Answer from the drawing. Dimensions are ordinates in mm from the lowest x, y and z of the part. A direction names the side the tool comes from. Coordinates: 2 decimals unless noted, no trailing zeros. Loops run counter-clockwise (first coordinate to the right, second up) from the corner with the lowest first, then second, coordinate; pieces in that order, holes last. Notation, with made-up numbers: M 18,-3 L 70,-3 A25 cw 70,19 Z; hole C 63,25.5 d1. An arc over 180 degrees is marked long. One line per item, written item: value. Start each with the question number.
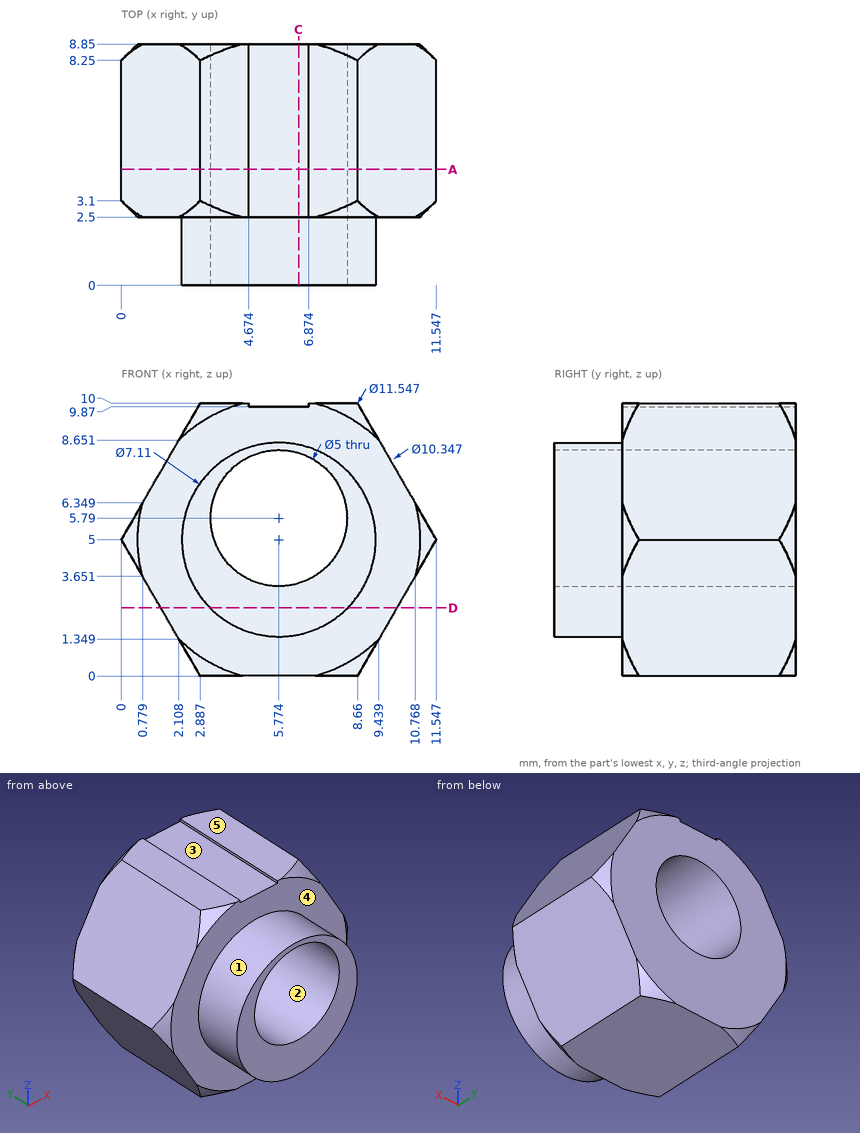
1) Flat-ended cylindrical pins translate along their axes: pin 1 (2 mm diameter, centred on x = 7.5, y = 1, fed in from +Z); pin 2 (1 mm diameter, centred on x = 2, y = 8, fed in from -Z); pin 3 (1.5 mm diameter, centred on y = 2.5, z = 5.5, fed in from +X); pin 4 (4.5 mm diameter, centred on x = 5.77, z = 5.79, fed in from -Y) (3 decimals). Find the tip coordinate at first contact, or state that the pin passes through.
2) A tool of negligible diameter and unlimited length cuts with its end or side. For the marked faces 4 and 5, from which of +Z, -Z, +X, -X, +Y, -Y can it reach the whole face along a straight path? Write none if from no direction.
3) For a pull along Z with two mould halves and no side action, classify the marked faces 1, 2 and 3 as released by +Z, released by -Z, zero draft, split by the parting line, or undercut.
4) Section A-A (y = 4.25) is taken. Determine the outline of the cut face in (x, z).
5) Consider line 1 along Y through (x, z) = (1.75, 4.25); line 2 along Z through (x, y) = (7.5, 1) (1 decimal); line 3 along Z through (x, y) = (7.5, 4.5). Determine where each line is inside the solid, lowest interval first.
6) Section D-D (z = 2.5) is taken. Determine the outline of the cut face in (x, y).
7) Section C-C (x = 6.5) is taken. Determine the outline of the cut face in (y, z).
Results found:
1. pin 1: stops at z = 8.48
1. pin 2: stops at z = 0.67
1. pin 3: stops at x = 11.53
1. pin 4: passes through
2. face 4: -Y
2. face 5: +Z, +X, -X, +Y, -Y
3. face 1: split by the parting line
3. face 2: undercut
3. face 3: released by +Z
4. outline: M 0,5 L 2.89,0 L 8.66,0 L 11.55,5 L 8.66,10 L 6.87,10 L 6.87,9.87 L 4.67,9.87 L 4.67,10 L 2.89,10 Z; hole C 5.77,5.79 d5
5. line 1: y = 2.5 to 8.85
5. line 2: z = 1.9 to 4, 7.6 to 8.1
5. line 3: z = 0 to 3.98, 7.6 to 10
6. outline: M 1.44,2.5 L 3.25,2.5 L 3.25,0 L 8.3,0 L 8.3,2.5 L 10.1,2.5 L 10.1,8.85 L 1.44,8.85 Z
7. outline: M 0,1.52 L 2.5,1.52 L 2.5,0 L 8.85,0 L 8.85,3.4 L 0,3.4 Z; M 0,8.18 L 8.85,8.18 L 8.85,9.87 L 2.5,9.87 L 2.5,8.48 L 0,8.48 Z
